Verification items for the finished model (mm, model axes). A direction names the side the tool comes from. Coordinates: 2 decimals unless noted, no trailing zeros. Order: outer loops, then holes, each group sorted by start corner. A loop starts at its lowest first (then second) coordinate and runs counter-clockwise, first axis right, second up. Notation, with made-up numbers: M 40.25,28 L 94.25,28 A26 ccw 94.25,59 Z; hole C -27.5,82 d1. An arc over 180 degrees is marked long. Answer as a JSON object with one key per item and string values. Group by question number.
(1) Cross-section at A-A (z = 0). Enter the section's corners in (x, y), plus the area to 3 significant figures.
(2) Cross-section at B-B (x = 0). Enter the section's corners in (y, z), plus the area to 3 significant figures.
(3) Access from +Z, -Z, +X, -X, +Y, -Y to the whole of each face (thin tool, end or side, straight path). Record for faces 1 (the face through (0, 4, 0)), 2 (the face through (0.66, 2.986, 14.985)), 3 (the face through (-12, -2, 12)).
(4) Cross-section at C-C (y = -1.25). Enter the section's corners in (x, z), plus the area to 3 significant figures.
(5) Material ranges on line 1 (Y direction, x = 12, z = 10.5); line 2 (X direction, y = 1.5, z = -4); line 3 (Z direction, x = -23.5, y = -0.25), recorded low to high.
(6) Gauge pin test, flat ends, axial feed: pin 1 Ø16.5 at (x, z) = (-13, -13.5) entering from +Y; pin 2 Ø8 at (x, z) = (23.5, -3.5) entering from -Y; pin 3 Ø2 at (y, z) = (-1.5, -20) entering from +X. Record the tip position at first contact, or that the pin passes through.
from build123d import *

# Parameters (mm, degrees)
BOSS_EXTRU_1_DEPTH      = 2
BOSS_EXTRU_1_DEPTH_BACK = 2
ESQUISSE1_R             = 30
CHANFREIN1_SIZE2        = 2.300736814
CHANFREIN1_SIZE         = 2
CHANFREIN2_SIZE         = 2.300736814
CHANFREIN2_SIZE_2       = 2
ESQUISSE2_R             = 15
BOSS_EXTRU_2_DEPTH      = 2


# Some blends are built 0.0001 mm under size
with BuildPart() as part:
    # Esquisse1 → Boss.-Extru.1 (new, two sides: drawn at the far end of the back side and taken through both)
    with BuildSketch(Plane(origin=(0, 0, 0), x_dir=(1, 0, 0), z_dir=(0, 1, 0)).offset(-BOSS_EXTRU_1_DEPTH_BACK)):
        with Locations(Location((0, 0, 0), (0, 0, 270))):
            Circle(ESQUISSE1_R)
    extrude(amount=BOSS_EXTRU_1_DEPTH + BOSS_EXTRU_1_DEPTH_BACK)

    # Chanfrein1
    chanfrein1_edges = [part.edges().sort_by_distance(p)[0] for p in [
        (0, 2, -30),
    ]]
    chanfrein1_side = [part.faces().sort_by_distance(p)[0] for p in [
        (0, 1.96, -30),
    ]]
    chamfer(chanfrein1_edges, length=CHANFREIN1_SIZE - 0.0001, length2=CHANFREIN1_SIZE2 - 0.0001, reference=chanfrein1_side[0])  # a hair under: the kernel refuses the full size

    # Chanfrein2
    # the kernel refuses this chamfer: 2.300736814, 2 mm, written as the material it takes off along each edge
    with BuildSketch(Plane(origin=(0, -2, 0), x_dir=(0, 0, 1), z_dir=(-1, 0, 0))) as chanfrein2_piece_1:
        Polygon((30, CHANFREIN2_SIZE), (30 - CHANFREIN2_SIZE_2, 0), (30, 0), align=None)
    revolve(axis=Axis((0, -2, 0), (0, 1, 0)), mode=Mode.SUBTRACT)

    # Esquisse2 → Boss.-Extru.2 (add)
    with BuildSketch(Plane.XZ.offset(2)):
        with Locations(Location((0, 0, 0), (0, 0, 270))):
            Circle(ESQUISSE2_R)
    boss_extru_2 = extrude(amount=BOSS_EXTRU_2_DEPTH)

    # Symétrie1: Boss.-Extru.2 across plane
    add(boss_extru_2.mirror(Plane.ZX))


solid = part.part
Taken from the geometry:
{
 "1": {"outline": "M -29.85,0.13 L -28,-2 L -15,-2 L -15,-4 L 15,-4 L 15,-2 L 28,-2 L 29.85,0.13 L 27.7,2 L 15,2 L 15,4 L -15,4 L -15,2 L -27.7,2 Z", "area": "351 mm²"},
 "2": {"outline": "M -4,-15 L -2,-15 L -2,-28 L 0.13,-29.85 L 2,-27.7 L 2,-15 L 4,-15 L 4,15 L 2,15 L 2,27.7 L 0.13,29.85 L -2,28 L -2,15 L -4,15 Z", "area": "351 mm²"},
 "3": {"face 1": "+Z, -Z, +X, -X, +Y", "face 2": "+Y", "face 3": "-Y"},
 "4": {"outline": "C 0,0 d57.3", "area": "2,580 mm²"},
 "5": {"line 1": "y = -2 to 2", "line 2": "x = -27.99 to 27.99", "line 3": "z = -17.87 to 17.87"},
 "6": {"pin 1": "stops at y = 4", "pin 2": "stops at y = -2", "pin 3": "stops at x = 21.73"}
}
